Design review of the part built by this model. Coordinates are the model's own, in mm. Face numbers are marked on the shaded views. A direction names the side the tool comes from. Round coordinates to 2 decimals unless told otherwise and drop trailing zeros. Order: outer loops, then holes, each group sorted by start corner. A loop starts at its lowest first (then second) coordinate and runs counter-clockwise, first axis right, second up. Notation, with made-up numbers: (-18, -12.75) - (30, -12.75) arc R24 cw to (30, 18.25) - close; hole circle Ø4 at (33.5, -23.5). An arc over 180 degrees is marked (long way). Use CSV: the item, a comma, the result in double quotes.
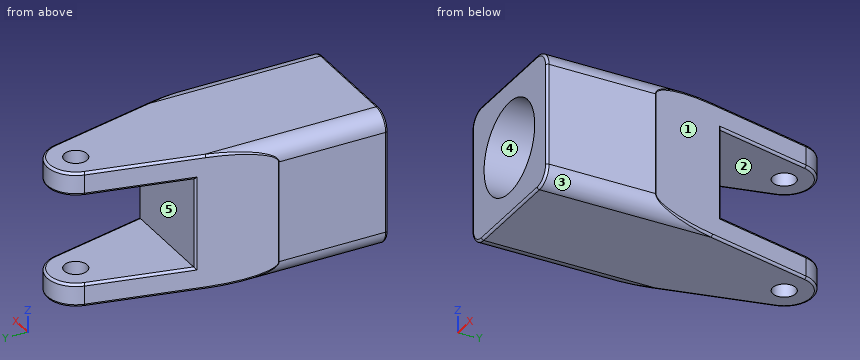
from build123d import *

# Parameters (mm, degrees)
EXTRUDE_1_DEPTH     = 9.5
EXTRUDE_2_DEPTH     = 11.8
EXTRUDE_3_DEPTH     = 2
CUT_EXTRUDE_1_REACH = 31.556
SKETCH_4_R          = 1.0000000000000002
FILLET_1_R          = 1.5
FILLET_2_R          = 0.2


with BuildPart() as part:
    # 草图1 → 凸台-拉伸1 (new body)
    with BuildSketch(Plane(origin=(0, 0, 0), x_dir=(1, 0, 0), z_dir=(0, 1, 0))):
        Polygon((5.899999999999999, 5.9), (5.9, -5.9), (-5.9, -5.900000000000002), (-5.900000000000002, 5.899999999999999), align=None)
    extrude(amount=EXTRUDE_1_DEPTH)

    # 草图2 → 凸台-拉伸2 (add)
    with BuildSketch(Plane.XY.offset(5.900000000000001)):
        Polygon((-5.900000000000001, 9.5), (5.8999999999999995, 9.5), (4.3999999999999995, 16), (-4.400000000000001, 16), align=None)
    extrude(amount=-EXTRUDE_2_DEPTH)

    # 草图3 → 凸台-拉伸3 (add)
    with BuildSketch(Plane.XY.offset(5.900000000000001)):
        with BuildLine():
            Line((-4.400000000000001, 16), (4.3999999999999995, 16))
            Line((4.3999999999999995, 16), (2.435977989236515, 24.510762046641762))
            ThreePointArc((2.435977989236515, 24.510762046641762), (-4.169e-14, 26.448613279894865), (-2.435977989236587, 24.510762046641744))
            Line((-2.435977989236587, 24.510762046641744), (-4.400000000000001, 16))
        make_face()
    extrude_3 = extrude(amount=-EXTRUDE_3_DEPTH)

    # 草图4 → 切除-拉伸1 (cut, up to next)
    with BuildSketch(Plane.XY.offset(5.900000000000001), mode=Mode.PRIVATE) as cut_extrude_1_sk1:
        with Locations((-3.296e-14, 23.948613279894865)):
            Circle(SKETCH_4_R)
    cut_extrude_1_tool1 = extrude(cut_extrude_1_sk1.sketch, amount=-CUT_EXTRUDE_1_REACH, mode=Mode.PRIVATE) & part.part
    cut_extrude_1 = cut_extrude_1_tool1.solids().sort_by_distance((0, 23.948613, 5.9))[0]
    add(cut_extrude_1, mode=Mode.SUBTRACT)

    # 镜向1: 凸台-拉伸3, 切除-拉伸1 across plane
    add(extrude_3.mirror(Plane.XY))
    add(cut_extrude_1.mirror(Plane.XY), mode=Mode.SUBTRACT)

    # 草图5 → 切除-旋转1 (revolve, cut)
    with BuildSketch(Plane.XY, mode=Mode.PRIVATE) as cut_revolve_1_sk:
        Polygon((0, 0), (0, 14), (3, 14), (3.999999999999999, 9.5), (4, 0), align=None)
    revolve(cut_revolve_1_sk.sketch.rotate(Axis((0, 0, 0), (0, 1, 0)), 90), axis=Axis((0, 0, 0), (0, 1, 0)), mode=Mode.SUBTRACT)

    # 圆角1
    fillet_1_edges = [part.edges().sort_by_distance(p)[0] for p in [
        (5.899999999999999, 4.75, -5.9),
        (5.9, 4.75, 5.9),
        (-5.9, 4.75, 5.900000000000002),
        (-5.900000000000002, 4.75, -5.899999999999999),
    ]]
    fillet(fillet_1_edges, radius=FILLET_1_R)

    # 圆角2
    fillet_2_edges = [part.edges().sort_by_distance(p)[0] for p in [
        (3.417988994618258, 20.25538102332088, 5.900000000000001),
        (5.19350478455585, 12.56147926692465, 5.672929753319866),
        (5.8999999999999995, 9.5, -8.9e-16),
        (5.193504784555849, 12.561479266924657, -5.672929753319866),
        (3.4179889946182564, 20.255381023320886, -5.9),
        (-4.254e-14, 26.448613279894865, -5.900000000000001),
        (-4.254e-14, 26.448613279894865, -3.9000000000000012),
        (-3.417988994618308, 20.255381023320872, -5.9),
        (-5.193504714374944, 12.561479571041913, -5.672929797068456),
        (-5.900000000000001, 9.5, 1.78e-15),
        (-5.193504714374941, 12.561479571041922, 5.672929797068459),
        (-3.4179889946183075, 20.255381023320876, 5.900000000000001),
        (0, 0, 5.900000000000001),
        (5.460660171779821, 0, 5.460660171779821),
        (5.8999999999999995, 0, 0),
        (5.4606601717798195, 0, -5.460660171779821),
        (-1.78e-15, 0, -5.8999999999999995),
        (-5.460660171779823, 0, -5.4606601717798195),
        (-5.900000000000001, 0, 1.78e-15),
        (-4.254e-14, 26.448613279894865, 5.900000000000001),
        (-4.254e-14, 26.448613279894865, 3.9000000000000012),
        (-5.460660171779821, 0, 5.460660171779823),
        (3.4179889946182582, 20.25538102332088, 3.9000000000000012),
        (-3.4179889946182938, 20.255381023320872, -3.9000000000000012),
        (3.4179889946182582, 20.25538102332088, -3.9000000000000012),
        (4.4, 16, 0),
        (-3.4179889946182933, 20.255381023320872, 3.9000000000000012),
        (-4.4, 16, 0),
    ]]
    fillet(fillet_2_edges, radius=FILLET_2_R)


solid = part.part
1) We need section A-A (x = 0). Give the number of separate pieces and of enclosed holes in the cut face, then the cut area to 3 significant figures.
Data:
separate pieces,"3"
enclosed holes,"0"
area,"115 mm2"
2) For the marked faces 1 and 2, list the 3-axis set-ups (+Z, -Z, +X, -X, +Y, -Y) from which the entire face can be reached by the end or side of a thin tool; tool diameter is ignored.
Data:
face 1,"+Z, -Z, +X, +Y"
face 2,"+X, -X, +Y"
3) Insertion check: pin 1 Ø3 at (y, z) = (19, 4.5) entering from -X; pin 2 Ø1.8 at (x, z) = (-0.5, -0.5) entering from -Y. Each pin has a flat end and moves straight along its axis. Give the tip position at first contact, or say it passes through.
Data:
pin 1,"stops at x = -4.05"
pin 2,"stops at y = 14"
4) To check wall thickness, follow L1, parallel to X at y = 5.5, z = 0; L2, parallel to Y at x = 0, z = -4.35; L3, parallel to Z at x = 2.75, y = 19.5. State the ranges of each line that lie inside material, in increasing order. Write a range as from..to.
Data:
L1,"x = -5.9..-4, 4..5.9"
L2,"y = 0..22.95, 24.95..26.45"
L3,"z = -5.9..-3.9, 3.9..5.9"
5) The part is to be moulded in two halves that separate along X. For the marked faces 3, 4 and 5, say which applies: +X half, -X half, draft (parallel to the pull), parting line (faces both ways), or undercut.
Data:
face 3,"+X half"
face 4,"undercut"
face 5,"draft"
6) We need section B-B (z = 0). Give the boundary of the cut face in (x, y), then the cut area to 3 significant figures.
Data:
outline,"(-5.9, 0.2) arc R0.2 ccw to (-5.7, 0) - (-4, 0) - (-4, 9.5) - (-3, 14) - (3, 14) - (4, 9.5) - (4, 0) - (5.7, 0) arc R0.2 ccw to (5.9, 0.2) - (5.9, 9.48) arc R0.2 ccw to (5.89, 9.52) - (4.44, 15.84) arc R0.2 ccw to (4.24, 16) - (-4.24, 16) arc R0.2 ccw to (-4.44, 15.84) - (-5.89, 9.52) arc R0.2 ccw to (-5.9, 9.48) - close"
area,"71.5 mm2"
